Source: CAD feature listing. Evaluate the final solid. Frame: model axes, mm. Face numbers are marked on the shaded views. A direction names the side the tool comes from. Coordinates: 2 decimals unless noted, no trailing zeros. Order: outer loops, then holes, each group sorted by start corner. A loop starts at its lowest first (then second) coordinate and runs counter-clockwise, first axis right, second up. Notation, with made-up numbers: (40.5, 24) -> (77.5, 24) arc R27 ccw to (77.5, 51) -> close; hole circle Ø6 at (22.5, 81.5). An arc over 180 degrees is marked (long way). Put each result on its own line as item: value.
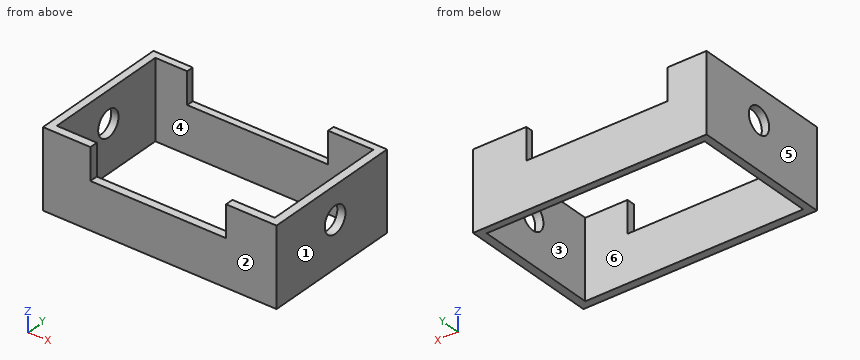
from build123d import *

# Parameters (mm, degrees)
F0_W     = 151.8262028694
F0_H     = 91.8187052011
F0_W_2   = 141.7044624686
F0_H_2   = 81.9379538298
F1_DEPTH = 50.8
F2_W     = 88.1531722844
F2_H     = 20.622967425
F3_DEPTH = 25.4
F4_R     = 8.6388854617
F5_DEPTH = 25.4
F6_R     = 8.4622870675
F7_DEPTH = 25.4
F8_W     = 91.5777124465
F8_H     = 20.5506539524
F9_DEPTH = 25.4


with BuildPart() as f1:
    # F0 (on Top) → F1 (new body)
    with BuildSketch(Plane.XY):
        with Locations((-0.12049824, -9.6397586167)):
            Rectangle(F0_W, F0_H)
        with Locations((-0.3614909947, -9.278267622)):
            Rectangle(F0_W_2, F0_H_2, mode=Mode.SUBTRACT)
    extrude(amount=F1_DEPTH)

    # F2 (on face) → F3 (cut)
    with BuildSketch(Plane.XZ.offset(55.5491112173)):
        with Locations((-1.130355522, 40.4885162875)):
            Rectangle(F2_W, F2_H)
    extrude(amount=-F3_DEPTH, mode=Mode.SUBTRACT)

    # F4 (on face) → F5 (cut)
    with BuildSketch(Plane.YZ.offset(75.7926031947)):
        with Locations((-6.8683284335, 29.7627560794)):
            Circle(F4_R)
    extrude(amount=-F5_DEPTH, mode=Mode.SUBTRACT)

    # F6 (on face) → F7 (cut)
    with BuildSketch(Plane.YZ.offset(-71.213722229)):
        with Locations((-7.3503162712, 30.4857380688)):
            Circle(F6_R)
    extrude(amount=-F7_DEPTH, mode=Mode.SUBTRACT)

    # F8 (on face) → F9 (cut)
    with BuildSketch(Plane(origin=(0, 36.2695939839, 0), x_dir=(-1, 0, 0), z_dir=(0, 1, 0))):
        with Locations((4.6993810683, 40.5246730238)):
            Rectangle(F8_W, F8_H)
    extrude(amount=-F9_DEPTH, mode=Mode.SUBTRACT)


solid = f1.part
1. Pull-direction query (Y, two-part tool) for the marked faces 1, 2, 3 and 4; classes: pulls with the +Y half, pulls with the -Y half, needs draft (parallel to the pull), parting line crosses it, or undercut.
Numbers:
face 1: needs draft
face 2: pulls with the -Y half
face 3: undercut
face 4: undercut
2. Cut plane A-A on x = -41. Output: boundary loops of the cut face in (y, z).
Numbers:
outline: (-55.55, 0) -> (-50.25, 0) -> (-50.25, 30.18) -> (-55.55, 30.18) -> close; (31.69, 0) -> (36.27, 0) -> (36.27, 30.25) -> (31.69, 30.25) -> close
3. First-contact query: pin 1 (5 mm diameter, centred on x = -18, y = 34.5, fed in from +Z). Flat tip, straight axial feed; report the tip coordinate or a pass-through.
Numbers:
pin 1: stops at z = 30.25
4. Cut plane B-B on y = -41. Output: boundary loops of the cut face in (x, z), plus the area to 3 significant figures.
Numbers:
outline: (-76.03, 0) -> (-71.21, 0) -> (-71.21, 50.8) -> (-76.03, 50.8) -> close; (70.49, 0) -> (75.79, 0) -> (75.79, 50.8) -> (70.49, 50.8) -> close
area: 514 mm2
5. Cut plane D-D on z = 33. Output: boundary loops of the cut face in (x, y), plus the area to 3 significant figures.
Numbers:
outline: (-76.03, -55.55) -> (-45.21, -55.55) -> (-45.21, -50.25) -> (-71.21, -50.25) -> (-71.21, -15.43) -> (-76.03, -15.43) -> close; (-76.03, 0.73) -> (-71.21, 0.73) -> (-71.21, 31.69) -> (-50.49, 31.69) -> (-50.49, 36.27) -> (-76.03, 36.27) -> close; (41.09, 31.69) -> (70.49, 31.69) -> (70.49, 1.14) -> (75.79, 1.14) -> (75.79, 36.27) -> (41.09, 36.27) -> close; (42.95, -55.55) -> (75.79, -55.55) -> (75.79, -14.88) -> (70.49, -14.88) -> (70.49, -50.25) -> (42.95, -50.25) -> close
area: 1,280 mm2
6. Set-up query: the marked faces 5 and 6. Return all of +Z, -Z, +X, -X, +Y, -Y with unobstructed straight access to the full face (end or side cutting, diameter ignored); none if empty.
Numbers:
face 5: +Z, -Z, -X, +Y, -Y
face 6: +Z, -Z
7. Ray query, line 1 along Y through (x, z) = (64.5, 24); line 2 along X through (y, z) = (-21, 47.5). Return the intervals inside material, ascending.
Numbers:
line 1: y = -55.55 to -50.25, 31.69 to 36.27
line 2: x = -76.03 to -71.21, 70.49 to 75.79
8. Cut plane C-C on z = 4.5. Output: boundary loops of the cut face in (x, y), plus the area to 3 significant figures.
Numbers:
outline: (-76.03, -55.55) -> (75.79, -55.55) -> (75.79, 36.27) -> (-76.03, 36.27) -> close; hole (-71.21, -50.25) -> (70.49, -50.25) -> (70.49, 31.69) -> (-71.21, 31.69) -> close
area: 2,330 mm2
